Source: three-view drawing plus pictorial views. Frame: mm from the lowest corner of the part. Coordinates: 2 decimals unless noted, no trailing zeros. Write each loop counter-clockwise with the first axis right and the second up, starting at its lowest first coordinate (ties: lowest second). Pieces come first, ordered by that corner, then holes. Notation, with made-up numbers: M 18.25,-4.5 L 35.25,-4.5 A27 ccw 35.25,20.5 Z; hole C -32.75,23.25 d11. An arc over 180 degrees is marked long. Write item = value, one per line. Start each with the question number.
Item 1: Section A-A on x = 3.25. Output: boundary loops of the cut face in (y, z), plus the area to 3 significant figures.
Item 2: First-contact query: pin 1 Ø1.5 at (x, y) = (4, 52) entering from +Z; pin 2 Ø10 at (x, z) = (5.5, 6.5) entering from +Y (3 decimals); pin 3 Ø6 at (x, z) = (7, 36) entering from -Y. Flat tips, straight axial feed; report the tip coordinate or a pass-through.
Item 3: Section B-B on z = 4. Output: boundary loops of the cut face in (x, y), plus the area to 3 significant figures.
Item 4: Ray query, L1, parallel to Z at x = 15.5, y = 19; L2, parallel to Z at x = 10.25, y = 31; L3, parallel to Y at x = 16.25, z = 31. Return the intervals inside material, ascending. Write a range as [from, to].
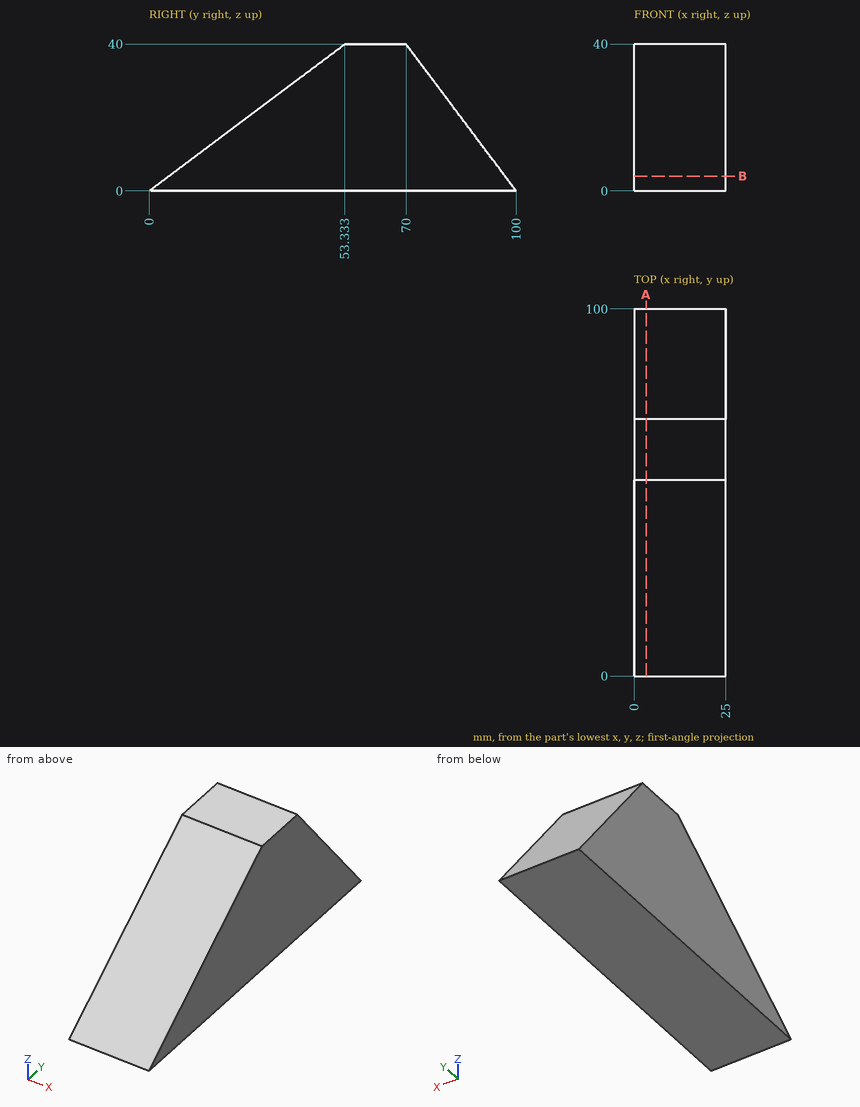
Responses:
q1.outline = M 0,0 L 100,0 L 70,40 L 53.33,40 Z
q1.area = 2,330 mm²
q2.pin_1 = 39.56
q2.pin_2 = 98.875
q2.pin_3 = 44
q3.outline = M 0,5.33 L 25,5.33 L 25,97 L 0,97 Z
q3.area = 2,290 mm²
q4.L1 = [0, 14.25]
q4.L2 = [0, 23.25]
q4.L3 = [41.33, 76.75]
